Input: part model. Units: mm. Frame: model coordinates. Face numbers are marked on the shaded views. A direction names the side the tool comes from. Round coordinates to 2 decimals unless told otherwise and drop trailing zeros. Loops run counter-clockwise (first coordinate to the right, second up) from the corner with the lowest first, then second, coordinate; pieces in that order, holes last. Notation, with made-up numbers: (-37, 37) - (-25, 37) arc R25 cw to (-25, 65) - close; hole circle Ø2 at (45, 66.5). An arc over 180 degrees is marked (long way). One line per question, with ' | ' between items. Start each with the question number.
Item 1: Section C-C, the plane x = 13.5. Return loops of the section in (y, z).
Item 2: Section A-A, the plane z = 0. Return loops of the section in (x, y).
Item 3: Material intervals for line 1 along Z through (x, y) = (12.25, 0); line 2 along X through (y, z) = (28, 17); line 3 along Z through (x, y) = (7.75, -8.5), sorted ascending.
Item 4: Set-up query: the marked faces 1 and 2. Return all of +Z, -Z, +X, -X, +Y, -Y with unobstructed straight access to the full face (end or side cutting, diameter ignored); none if empty.
Item 5: Draft query along Y for the marked faces 3, 4 and 5. Return one class per face: pulls with the +Y half, pulls with the -Y half, needs draft (parallel to the pull), parting line crosses it, or undercut.
Item 6: First-contact query: pin 1 (12 mm diameter, centred on x = 15.5, y = -10.5, fed in from +Z); pin 2 (6 mm diameter, centred on x = 13, z = 1, fed in from +Y); pin 3 (3 mm diameter, centred on x = 14, y = 19, fed in from -Z). Flat tips, straight axial feed; report the tip coordinate or a pass-through.
Item 7: Section D-D, the plane y = -32. Return loops of the section in (x, z).
```python
from build123d import *

# Parameters (mm, degrees)
RADYUS1_R = 5


with BuildPart() as part:
    # Çizim1 → Döndür1 (revolve)
    with BuildSketch(Plane.XY):
        Polygon((0, 37.5), (2, 37.5), (2, 20), (20, 20), (20, 15), (0, 15), align=None)
    revolve(axis=Axis((0, 0, 0), (1, 0, 0)))

    # Radyus1
    radyus1_edges = [part.edges().sort_by_distance(p)[0] for p in [
        (2, -20, 0),
    ]]
    fillet(radyus1_edges, radius=RADYUS1_R)


solid = part.part
```
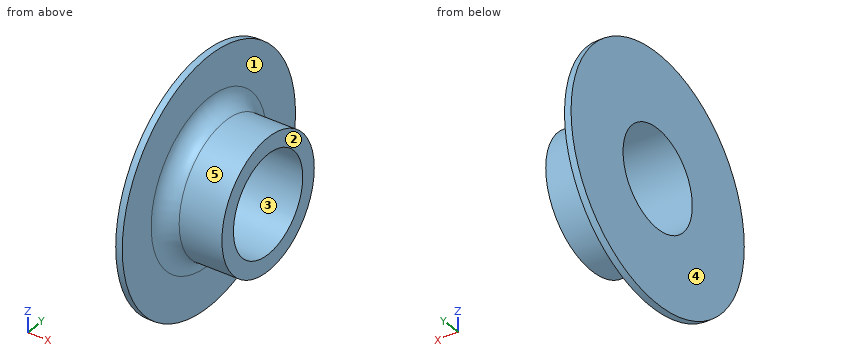
Return value:
1) outline: circle Ø40 at (0, 0); hole circle Ø30 at (0, 0)
2) outline: (0, -37.5) - (2, -37.5) - (2, -25) arc R5 cw to (7, -20) - (20, -20) - (20, -15) - (0, -15) - close; (0, 15) - (20, 15) - (20, 20) - (7, 20) arc R5 cw to (2, 25) - (2, 37.5) - (0, 37.5) - close
3) line 1: -20 to -15, 15 to 20 | line 2: 0 to 2 | line 3: -18.1 to -12.36, 12.36 to 18.1
4) face 1: +X | face 2: +Z, -Z, +X, +Y, -Y
5) face 3: undercut | face 4: needs draft | face 5: parting line crosses it
6) pin 1: z = 19.49 | pin 2: y = 20 | pin 3: z = -9.68
7) outline: (0, -19.55) - (2, -19.55) - (2, 19.55) - (0, 19.55) - close
